Can you work these out from the model? Positions are in its coordinate system, mm. Face numbers are marked on the shaded views. A direction names the side the tool comes from. Round coordinates to 2 decimals unless told otherwise and drop trailing zeros. Write each loop counter-clockwise with the first axis right and the second up, starting at its lowest first coordinate (ties: lowest second). Pieces come first, ordered by that corner, then holes. Notation, with made-up numbers: M -19,-8.75 L 22,-8.75 A22 ccw 22,13.25 Z; hole C 49.5,77.5 d2. An arc over 180 degrees is marked long. Answer as a JSON object with one key per item and string values. Group by question number.
1) I'm going to push flat-ended pins straight in: pin 1 Ø4 at (x, z) = (0, 25.18) entering from +Y; pin 2 Ø8 at (x, y) = (0.5, 5) entering from +Z; pin 3 Ø4 at (x, y) = (0.5, 6.5) entering from -Z; pin 4 Ø6 at (x, z) = (-4, 18) entering from +Y. Where does each tip first touch, or does it pass through?
2) On a 3-axis mill with a long thin cutter (end or side, diameter ignored), from which of +Z, -Z, +X, -X, +Y, -Y can I reach the whole of each face in a straight line? I mean the marked faces 4, 5 and 6. Say none if no direction works.
3) Suppose I cut it at B-B, the plane x = 5. Write out the boundary of the cut face in (y, z).
4) Suppose I cut it at A-A, the plane y = 12.5. Write out the boundary of the cut face in (x, z), and give its area (3 significant figures).
5) Suppose I cut it at C-C, the plane z = 18. Write out the boundary of the cut face in (x, y).
6) Please list where these lines run through material, in increasing order: L1, parallel to X at y = -2.25, z = 9; L2, parallel to X at y = 2, z = 32; L3, parallel to Z at x = 0.5, y = -6. Write a range as [from, to].
7) If we mould it in two halves opening along X, with no side actions, what happens to the marked faces 1, 2 and 3? For each: +X half, -X half, draft (parallel to the pull), parting line (faces both ways), or undercut.
8) Suppose I cut it at D-D, the plane x = -6. Write out the boundary of the cut face in (y, z).
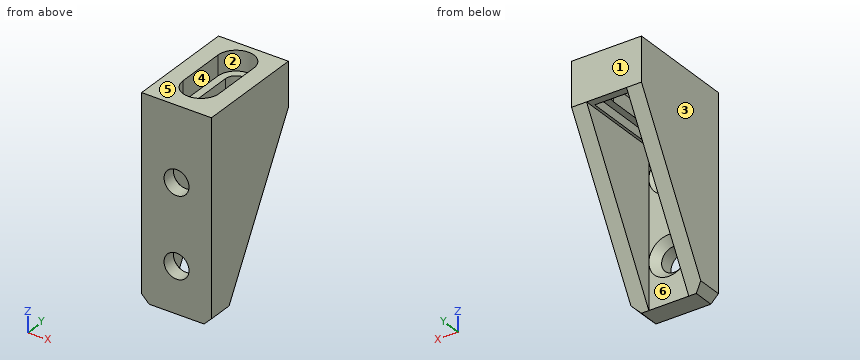
from build123d import *

# Parameters (mm, degrees)
SALIENTE_EXTRUIR1_DEPTH = 40
CORTAR_EXTRUIR1_DEPTH   = 4
CORTAR_EXTRUIR2_DEPTH   = 45.955533586
CROQUIS4_W              = 8
CROQUIS4_H              = 31.180864131
CORTAR_EXTRUIR3_DEPTH   = 17.81659
CROQUIS5_W              = 6.9
CROQUIS5_H              = 16.9
CORTAR_EXTRUIR4_DEPTH   = 1.819135869
CROQUIS6_R              = 2.5
CORTAR_EXTRUIR5_DEPTH   = 45.34445566
CHAFL_N1_SIZE           = 1.5
CHAFL_N2_SIZE           = 1.5


with BuildPart() as part:
    # Croquis1 → Saliente-Extruir1 (new body)
    with BuildSketch(Plane.XY):
        Polygon((-7, 7), (-7, 15), (7, 15), (7, 7), (7, -7), (-7, -7), align=None)
        with BuildLine():
            Line((-2.1, 0), (-2.1, 10))
            ThreePointArc((-2.1, 10), (0, 12.1), (2.1, 10))
            Line((2.1, 10), (2.1, 0))
            ThreePointArc((2.1, 0), (0, -2.1), (-2.1, 0))
        make_face(mode=Mode.SUBTRACT)
    extrude(amount=SALIENTE_EXTRUIR1_DEPTH)

    # Croquis2 → Cortar-Extruir1 (cut)
    with BuildSketch(Plane.XY.offset(40)):
        with BuildLine():
            Line((-3.6, 0), (-3.6, 10))
            ThreePointArc((-3.6, 10), (0, 13.6), (3.6, 10))
            Line((3.6, 10), (3.6, 0))
            ThreePointArc((3.6, 0), (0, -3.6), (-3.6, 0))
        make_face()
    extrude(amount=-CORTAR_EXTRUIR1_DEPTH, mode=Mode.SUBTRACT)

    # Croquis3 → Cortar-Extruir2 (cut, through all)
    with BuildSketch(Plane(origin=(7, 0, 0), x_dir=(0, 0, -1), z_dir=(1, 0, 0))):
        Polygon((0, 15), (-31.180864131, 15), (0, -2.81658631), align=None)
    extrude(amount=-CORTAR_EXTRUIR2_DEPTH, mode=Mode.SUBTRACT)

    # Croquis4 → Cortar-Extruir3 (cut)
    with BuildSketch(Plane(origin=(0, 15, 0), x_dir=(1, 0, 0), z_dir=(0, 1, 0))):
        with Locations((0, -15.590432066)):
            Rectangle(CROQUIS4_W, CROQUIS4_H)
    extrude(amount=-CORTAR_EXTRUIR3_DEPTH, mode=Mode.SUBTRACT)

    # Croquis5 → Cortar-Extruir4 (cut)
    with BuildSketch(Plane(origin=(0, 0, 31.180864131), x_dir=(-1, 0, 0), z_dir=(0, 0, -1))):
        with Locations((0, 5)):
            Rectangle(CROQUIS5_W, CROQUIS5_H)
    extrude(amount=-CORTAR_EXTRUIR4_DEPTH, mode=Mode.SUBTRACT)

    # Croquis6 → Cortar-Extruir5 (cut, through all)
    with BuildSketch(Plane(origin=(0, -2.81658631, 0), x_dir=(1, 0, 0), z_dir=(0, 1, 0))):
        with Locations(Location((0, -9.180864131, 0), (0, 0, 270))):
            Circle(CROQUIS6_R)
        with Locations(Location((0, -25.180864131, 0), (0, 0, 270))):
            Circle(CROQUIS6_R)
    extrude(amount=-CORTAR_EXTRUIR5_DEPTH, mode=Mode.SUBTRACT)

    # Chaflán1
    chafl_n1_edges = [part.edges().sort_by_distance(p)[0] for p in [
        (0, -2.81659, 6.680864131),
        (0, -2.81659, 22.680864131),
    ]]
    chamfer(chafl_n1_edges, length=CHAFL_N1_SIZE - 0.0001)  # a hair under: the kernel refuses the full size

    # Chaflán2
    chafl_n2_edges = [part.edges().sort_by_distance(p)[0] for p in [
        (-7, -4.908293155, 0),
        (7, -4.908293155, 0),
    ]]
    chamfer(chafl_n2_edges, length=CHAFL_N2_SIZE)


solid = part.part
Results:
{
 "1": {"pin 1": "through", "pin 2": "z = 40", "pin 3": "z = 33", "pin 4": "y = 9.18"},
 "2": {"face 4": "+Z", "face 5": "+Z, +X, -X, +Y, -Y", "face 6": "-Z, +Y"},
 "3": {"outline": "M -7,0 L -2.82,0 L 15,31.18 L 15,40 L -7,40 Z"},
 "4": {"outline": "M -7,26.81 L -4,26.81 L -4,31.18 L -3.45,31.18 L -3.45,33 L 3.45,33 L 3.45,31.18 L 4,31.18 L 4,26.81 L 7,26.81 L 7,40 L 2.59,40 L 2.59,36 L -2.59,36 L -2.59,40 L -7,40 Z", "area": "116 mm^2"},
 "5": {"outline": "M -7,-7 L 7,-7 L 7,7.47 L 4,7.47 L 4,-2.82 L -4,-2.82 L -4,7.47 L -7,7.47 Z"},
 "6": {"L1": "[-7, -4], [4, 7]", "L2": "[-7, -3.45], [3.45, 7]", "L3": "[0, 6.73], [11.63, 22.73], [27.63, 40]"},
 "7": {"face 1": "draft", "face 2": "undercut", "face 3": "-X half"},
 "8": {"outline": "M -7,0.5 L -2.53,0.5 L 15,31.18 L 15,40 L -7,40 Z"}
}
